```python
from build123d import *

# Parameters (mm, degrees)
SKETCH1_R            = 254
SKETCH1_R_2          = 239
BOSS_EXTRUDE1_DEPTH  = 3.175
M3_CLEARANCE_HOLE1_D = 3.4


with BuildPart() as part:
    # Sketch1 → Boss-Extrude1 (new, symmetric)
    with BuildSketch(Plane(origin=(0, 0, 0), x_dir=(1, 0, 0), z_dir=(0, 1, 0))):
        with Locations(Location((0, 0, 0), (0, 0, 270))):
            Circle(SKETCH1_R)
        with Locations(Location((0, 0, 0), (0, 0, 270))):
            Circle(SKETCH1_R_2, mode=Mode.SUBTRACT)
    extrude(amount=BOSS_EXTRUDE1_DEPTH, both=True)

    # M3 Clearance Hole1 (through all)
    with Locations(Plane(origin=(0, 3.175, 0), x_dir=(1, 0, 0), z_dir=(0, 1, 0))):
        with Locations((248, 0), (243.23474954, -48.38239986), (229.122124063, -94.905491227), (206.204463851, -137.781417789), (175.362481734, -175.362481734), (137.781417789, -206.204463851), (94.905491227, -229.122124063), (48.38239986, -243.23474954), (0, -248), (-48.38239986, -243.23474954), (-94.905491227, -229.122124063), (-137.781417789, -206.204463851), (-175.362481734, -175.362481734), (-206.204463851, -137.781417789), (-229.122124063, -94.905491227), (-243.23474954, -48.38239986), (-248, 0), (-243.23474954, 48.38239986), (-229.122124063, 94.905491227), (-206.204463851, 137.781417789), (-175.362481734, 175.362481734), (-137.781417789, 206.204463851), (-94.905491227, 229.122124063), (-48.38239986, 243.23474954), (0, 248), (48.38239986, 243.23474954), (94.905491227, 229.122124063), (137.781417789, 206.204463851), (175.362481734, 175.362481734), (206.204463851, 137.781417789), (229.122124063, 94.905491227), (243.23474954, 48.38239986)):
            Hole(M3_CLEARANCE_HOLE1_D / 2)


solid = part.part
```
The model under review builds one solid part; all positions refer to its coordinate system, in mm. Round coordinates to 2 decimals unless told otherwise and drop trailing zeros. Write each loop counter-clockwise with the first axis right and the second up, starting at its lowest first coordinate (ties: lowest second). Pieces come first, ordered by that corner, then holes.
(1) Mouldability with a two-part tool opening along Z and no side actions: class faces 1 (the cylindrical face through (-247.96, 0.04, -55.06)), 2 (the flat face through (-149.3, -3.175, 187)), 3 (the cylindrical face through (-91.538, -0.044, 220.775)) as +Z half, -Z half, draft (parallel to the pull), parting line (faces both ways), or undercut.
(2) We need section B-B on x = 161.5. Give the boundary of the cut face in (y, z) (3 decimals).
(3) We need section A-A on z = 220.5. Give the boundary of the cut face in (x, y) (3 decimals), and give its area (3 significant figures).
(4) Insertion check: pin 1 (5.5 mm diameter, centred on x = -206.2, z = -137.78, fed in from +Y) (3 decimals); pin 2 (1 mm diameter, centred on x = -112.5, y = 2, fed in from +Z); pin 3 (3 mm diameter, centred on x = 105, y = 1.5, fed in from -Z); pin 4 (3 mm diameter, centred on y = 0.5, z = 133.5, fed in from -X). Each pin has a flat end and moves straight along its axis. Give the tip position at first contact, or say it passes through.
(5) Wall thickness on L1, parallel to Z at x = 175, y = -1.5; L2, parallel to X at y = -2, z = -159; L3, parallel to Z at x = -181.5, y = 1.5: over which ranges is each line inside the solid? List them lowest first.
(6) We need section C-C on y = -0.5. Give the number of separate pieces and of enclosed holes in the cut face, and give its area (3 significant figures).
Findings below:
1. face 1: parting line
1. face 2: draft
1. face 3: undercut
2. outline: (-3.175, -196.045) - (3.175, -196.045) - (3.175, -176.178) - (-3.175, -176.178) - close; (-3.175, 176.178) - (3.175, 176.178) - (3.175, 196.045) - (-3.175, 196.045) - close
3. outline: (-126.078, -3.175) - (-92.2, -3.175) - (-92.2, 3.175) - (-126.078, 3.175) - close; (92.2, -3.175) - (126.078, -3.175) - (126.078, 3.175) - (92.2, 3.175) - close
3. area: 430 mm2
4. pin 1: stops at y = 3.175
4. pin 2: stops at z = 227.97
4. pin 3: stops at z = -231.96
4. pin 4: stops at x = -217.01
5. L1: z = -184.1 to -177.02, -173.7 to -162.78, 162.78 to 173.7, 177.02 to 184.1
5. L2: x = -198.08 to -178.44, 178.44 to 198.08
5. L3: z = -177.69 to -155.5, 155.5 to 177.69
6. separate pieces: 1
6. enclosed holes: 33
6. area: 22,900 mm2
